```python
from build123d import *

# Parameters (mm, degrees)
F0_W     = 28
F0_H     = 25
F1_DEPTH = 4
F2_W     = 25
F2_H     = 25
F3_DEPTH = 4
F5_D     = 2.4


with BuildPart() as f1:
    # F0 (on Top) → F1 (new body)
    with BuildSketch(Plane.XY):
        Rectangle(F0_W, F0_H)
    extrude(amount=-F1_DEPTH)

    # F2 (on Top) → F3 (join)
    with BuildSketch(Plane.XY):
        Rectangle(F2_W, F2_H)
    extrude(amount=F3_DEPTH)

    # F5 (through all)
    with Locations(Plane.XY.offset(4)):
        with Locations((-10, 10), (10, 10), (10, -10), (-10, -10)):
            Hole(F5_D / 2)


solid = f1.part
```
Geometry check sheet. Reference: the model listing, model coordinates, mm. A direction names the side the tool comes from. Give positions to 0.01 mm unless a question says otherwise; leave off trailing zeros. Loops run counter-clockwise (first coordinate to the right, second up) from the corner with the lowest first, then second, coordinate; pieces in that order, holes last. Notation, with made-up numbers: M -20.5,11.5 L -16.5,11.5 A9 cw -16.5,28.5 Z; hole C -33.75,55 d9. An arc over 180 degrees is marked long. Write item = value, one per line.
(1) Sectioned sample at C-C, the plane z = -3. Record the cut outline in (x, y), plus the area to 3 significant figures.
Answer below:
outline = M -14,-12.5 L 14,-12.5 L 14,12.5 L -14,12.5 Z; hole C -10,-10 d2.4; hole C -10,10 d2.4; hole C 10,-10 d2.4; hole C 10,10 d2.4
area = 682 mm2
(2) Tool access check on faces 5 (the face through (-12.5, 0, 2)), 6 (the face through (12.5, 0, 2)), 7 (the face through (0, 0, -4)). Record the directions out of +Z, -Z, +X, -X, +Y, -Y that give a thin tool (end or side, any length) a straight path to the whole face; none if there is none.
Answer below:
face_5 = +Z, -X, +Y, -Y
face_6 = +Z, +X, +Y, -Y
face_7 = -Z, +X, -X, +Y, -Y
(3) Material ranges on line 1 (Y direction, x = 10, z = 1.5); line 2 (X direction, y = -10.75, z = 3.5); line 3 (X direction, y = -10.5, z = 3), recorded low to high. Write a range as [from, to].
Answer below:
line_1 = [-12.5, -11.2], [-8.8, 8.8], [11.2, 12.5]
line_2 = [-12.5, -10.94], [-9.06, 9.06], [10.94, 12.5]
line_3 = [-12.5, -11.09], [-8.91, 8.91], [11.09, 12.5]
(4) Release check for a two-part mould opening along X. For faces 1 (the face through (9.446, 8.935, -0.056)), 2 (the face through (0, 12.5, 0)), 3 (the face through (14, 0, -2)), 4 (the face through (-9.74, -11.17, -0.06)) record: released by +X, released by -X, zero draft, split by the parting line, or undercut.
Answer below:
face_1 = undercut
face_2 = zero draft
face_3 = released by +X
face_4 = undercut
(5) Sectioned sample at B-B, the plane y = -10. Record the cut outline in (x, z), plus the area to 3 significant figures.
Answer below:
outline = M -14,-4 L -11.2,-4 L -11.2,4 L -12.5,4 L -12.5,0 L -14,0 Z; M -8.8,-4 L 8.8,-4 L 8.8,4 L -8.8,4 Z; M 11.2,-4 L 14,-4 L 14,0 L 12.5,0 L 12.5,4 L 11.2,4 Z
area = 174 mm2
(6) Sectioned sample at A-A, the plane x = 10. Record the cut outline in (y, z).
Answer below:
outline = M -12.5,-4 L -11.2,-4 L -11.2,4 L -12.5,4 Z; M -8.8,-4 L 8.8,-4 L 8.8,4 L -8.8,4 Z; M 11.2,-4 L 12.5,-4 L 12.5,4 L 11.2,4 Z
(7) Gauge pin test, flat ends, axial feed: pin 1 Ø0.8 at (x, y) = (-13, -4.5) entering from +Z; pin 2 Ø1.9 at (x, y) = (10, 10) entering from -Z; pin 3 Ø4.5 at (y, z) = (-5.5, 2.5) entering from -X. Record the tip position at first contact, or that the pin passes through.
Answer below:
pin_1 = 0
pin_2 = through
pin_3 = -12.5
(8) Sectioned sample at D-D, the plane y = -6.75. Record the cut outline in (x, z), plus the area to 3 significant figures.
Answer below:
outline = M -14,-4 L 14,-4 L 14,0 L 12.5,0 L 12.5,4 L -12.5,4 L -12.5,0 L -14,0 Z
area = 212 mm2
